Geometry check sheet. Reference: the model listing, model coordinates, mm. Round coordinates to 2 decimals unless told otherwise and drop trailing zeros. Order: outer loops, then holes, each group sorted by start corner. A loop starts at its lowest first (then second) coordinate and runs counter-clockwise, first axis right, second up.
(1) Cross-section at A-A on x = 20. Enter the section's corners in (y, z), and give its area (3 significant figures).
(2) Cross-section at B-B on y = 2.5. Enter the section's corners in (x, z), and give its area (3 significant figures).
(3) Thickness scan on L1, parallel to X at y = 7.25, z = 4; L2, parallel to X at y = 8.5, z = 5; L3, parallel to Z at x = 36.5, y = 1.5. Record the ranges inside material, lowest first.
(4) Draft check along Z on faces 1 (the face through (1.94, 5.07, 15.99)), 2 (the face through (20, 5, 40)), 3 (the face through (0, 5, 20)), 4 (the face through (34.67, 5.07, 4.69)). Enter one of: pulls with the +Z half, pulls with the -Z half, needs draft (parallel to the pull), parting line crosses it, or undercut.
(5) Cross-section at C-C on z = 37. Enter the section's corners in (x, y), and give its area (3 significant figures).
(6) Cross-section at D-D on x = 36. Enter the section's corners in (y, z), and give its area (3 significant figures).
from build123d import *

# Parameters (mm, degrees)
SKETCH1_W           = 40
SKETCH1_H           = 40
BOSS_EXTRUDE1_DEPTH = 10
SKETCH2_R           = 1.5
CUT_EXTRUDE1_DEPTH  = 58.445626465
SKETCH3_R           = 18.5
CUT_EXTRUDE2_DEPTH  = 10


with BuildPart() as part:
    # Sketch1 → Boss-Extrude1 (new body)
    with BuildSketch(Plane(origin=(0, 0, 0), x_dir=(1, 0, 0), z_dir=(0, 1, 0))):
        with Locations((20, -20)):
            Rectangle(SKETCH1_W, SKETCH1_H)
    extrude(amount=BOSS_EXTRUDE1_DEPTH)

    # Sketch2 → Cut-Extrude1 (cut, through all)
    with BuildSketch(Plane(origin=(0, 10, 0), x_dir=(1, 0, 0), z_dir=(0, 1, 0))):
        with Locations(Location((4, -36, 0), (0, 0, 270))):
            Circle(SKETCH2_R)
        with Locations(Location((36, -36, 0), (0, 0, 270))):
            Circle(SKETCH2_R)
        with Locations(Location((36, -4, 0), (0, 0, 270))):
            Circle(SKETCH2_R)
        with Locations(Location((4, -4, 0), (0, 0, 270))):
            Circle(SKETCH2_R)
    extrude(amount=-CUT_EXTRUDE1_DEPTH, mode=Mode.SUBTRACT)

    # Sketch3 → Cut-Extrude2 (cut)
    with BuildSketch(Plane(origin=(0, 10, 0), x_dir=(1, 0, 0), z_dir=(0, 1, 0))):
        with Locations(Location((20, -20, 0), (0, 0, 270))):
            Circle(SKETCH3_R)
    extrude(amount=-CUT_EXTRUDE2_DEPTH, mode=Mode.SUBTRACT)


solid = part.part
Found:
1. outline: (0, 0) - (10, 0) - (10, 1.5) - (0, 1.5) - close; (0, 38.5) - (10, 38.5) - (10, 40) - (0, 40) - close
1. area: 30.0 mm2
2. outline: (0, 0) - (40, 0) - (40, 40) - (0, 40) - close; hole circle Ø37 at (20, 20); hole circle Ø3 at (4, 4); hole circle Ø3 at (4, 36); hole circle Ø3 at (36, 4); hole circle Ø3 at (36, 36)
2. area: 497 mm2
3. L1: x = 0 to 2.5, 5.5 to 10.71, 29.29 to 34.5, 37.5 to 40
3. L2: x = 0 to 2.88, 5.12 to 9.17, 30.83 to 34.88, 37.12 to 40
3. L3: z = 0 to 2.59, 5.41 to 11.63, 28.37 to 34.59, 37.41 to 40
4. face 1: undercut
4. face 2: pulls with the +Z half
4. face 3: needs draft
4. face 4: undercut
5. outline: (0, 0) - (2.88, 0) - (2.88, 10) - (0, 10) - close; (5.12, 0) - (12.7, 0) - (12.7, 10) - (5.12, 10) - close; (27.3, 0) - (34.88, 0) - (34.88, 10) - (27.3, 10) - close; (37.12, 0) - (40, 0) - (40, 10) - (37.12, 10) - close
5. area: 209 mm2
6. outline: (0, 0) - (10, 0) - (10, 2.5) - (0, 2.5) - close; (0, 5.5) - (10, 5.5) - (10, 10.71) - (0, 10.71) - close; (0, 29.29) - (10, 29.29) - (10, 34.5) - (0, 34.5) - close; (0, 37.5) - (10, 37.5) - (10, 40) - (0, 40) - close
6. area: 154 mm2
